Read the model definition and answer for the solid it produces. Units are mm, in the model's axes. A direction names the side the tool comes from. Give positions to 0.01 mm unless a question says otherwise; leave off trailing zeros. Write each loop counter-clockwise with the first axis right and the second up, starting at its lowest first coordinate (ties: lowest second). Pieces come first, ordered by that corner, then holes. Notation, with made-up numbers: (-19.75, -37) - (37.25, -37) arc R12 ccw to (37.25, -14) - close; hole circle Ø9 at (-28.75, 81). An arc over 180 degrees is marked (long way). Answer as CSV lines item,"result".
Autodesk Inventor part; units mm, degrees
ref_plane "YZ Plane" through (0, 0, 0) normal (1, 0, 0) x (0, 1, 0)
ref_plane "XZ Plane" through (0, 0, 0) normal (0, 1, 0) x (-1, 0, 0)
ref_plane "XY Plane" through (0, 0, 0) normal (0, 0, 1) x (1, 0, 0)
sketch "Sketch1" plane through (0, 0, 0) normal (0, 0, 1) x (1, 0, 0)
  line L0 (0, 0) -> (76.2, 0)
  line L1 (76.2, 0) -> (76.2, 127)
  line L2 (76.2, 127) -> (0, 127)
  line L3 (0, 127) -> (0, 0)
  dimension "d0" = 76.2
  dimension "d1" = 127
extrude "Extrusion1" add sketch "Sketch1" along normal blind 25.4
sketch "Sketch2" plane through (76.2, 0, 0) normal (1, 0, 0) x (0, 0, -1)
  line L0 (0, 0) -> (-25.4, 0)
  line L1 (0, 0) -> (0, 127)
  line L2 (0, 127) -> (-25.4, 127)
  line L3 (0, 25.4) -> (-12.7, 25.4)
  line L4 (-12.7, 25.4) -> (-12.7, 101.6)
  line L5 (-12.7, 101.6) -> (0, 101.6)
  line L6 (0, 101.6) -> (0, 25.4)
  dimension "d4" = 12.7
  dimension "d5" = 25.4
  dimension "d6" = 25.4
extrude "Extrusion2" cut sketch "Sketch2" against normal through all
sketch "Sketch3" plane through (76.2, 0, 25.4) normal (1, 0, 0) x (0, 0, -1)
  line L0 (0, 127) -> (0, 0)
  line L1 (0, 88.9) -> (-12.7, 88.9)
  line L2 (-12.7, 88.9) -> (-12.7, 101.6)
  line L3 (-12.7, 101.6) -> (0, 101.6)
  line L4 (0, 101.6) -> (0, 88.9)
  line L5 (25.4, 127) -> (0, 127)
  dimension "d9" = 12.7
  dimension "d10" = 12.7
  dimension "d14" = 25.4
extrude "Extrusion3" add sketch "Sketch3" against normal up to surface (76.2 mm away) from surface at 0
equation "\"d6\" = d5"
properties part number "Slider"
(1) For faces 1 (the flat face through (39, 101.6, 32)), 2 (the flat face through (0, 64, 15)), 3 (the flat face through (39, 25.4, 6)), 4 (the flat face through (38, 45, 25.4)), determine the directions among +Z, -Z, +X, -X, +Y, -Y from which every point of the face is accessible in a straight line to the end or side of a thin tool.
Worked out:
face 1,"+Z, +X, -X, +Y"
face 2,"+Z, -Z, -X, +Y, -Y"
face 3,"-Z, +X, -X"
face 4,"+Z, +X, -X, -Y"
(2) A cutting plane is placed at C-C (z = 34). Write down the section's boundary in (x, y).
Worked out:
outline,"(0, 88.9) - (76.2, 88.9) - (76.2, 101.6) - (0, 101.6) - close"
(3) A cutting plane is placed at A-A (x = 39.5). Write down the section's boundary in (y, z).
Worked out:
outline,"(0, 0) - (25.4, 0) - (25.4, 12.7) - (101.6, 12.7) - (101.6, 0) - (127, 0) - (127, 25.4) - (101.6, 25.4) - (101.6, 38.1) - (88.9, 38.1) - (88.9, 25.4) - (0, 25.4) - close"
(4) A cutting plane is placed at B-B (y = 31). Write down the section's boundary in (x, z).
Worked out:
outline,"(0, 12.7) - (76.2, 12.7) - (76.2, 25.4) - (0, 25.4) - close"
(5) Find the intervals of material crossed by L1, parallel to Y at x = 53.5, z = 9.5; L2, parallel to Y at x = 58, z = 28.5; L3, parallel to Z at x = 56, y = 91, in increasing order.
Worked out:
L1,"y = 0 to 25.4, 101.6 to 127"
L2,"y = 88.9 to 101.6"
L3,"z = 12.7 to 38.1"
(6) Each of these flat-tipped pins is pushed along its axis until it touches: P1, Ø20.5, axis at x = 38, y = 120.5, coming from the +Z side; P2, Ø23, axis at x = 53, y = 59, coming from the -Z side; P3, Ø8, axis at x = 27.5, z = 31, coming from the -Y side; P4, Ø1.5, axis at y = 106.5, z = 27, coming from the +X side. Where does it stop, or does it pass through?
Worked out:
P1,"stops at z = 25.4"
P2,"stops at z = 12.7"
P3,"stops at y = 88.9"
P4,"passes through"
